Geometry: final body of the model. Coordinates: model frame, mm. A direction names the side the tool comes from. Round coordinates to 2 decimals unless told otherwise and drop trailing zeros. Loops run counter-clockwise (first coordinate to the right, second up) from the corner with the lowest first, then second, coordinate; pieces in that order, holes last. Notation, with made-up numbers: (26, 14) -> (30, 14) arc R17 ccw to (30, 20) -> close; hole circle Ø1 at (25.25, 14). An arc over 180 degrees is marked (long way). Answer in a Markdown table with one row per item.
```python
from build123d import *

# Parameters (mm, degrees)
F0_R     = 12.7
F0_R_2   = 9.525
F1_DEPTH = 50.8
F2_R     = 12.7
F4_DEPTH = 25.4
F3_R     = 9.525
F5_DEPTH = 25.4


with BuildPart() as f1:
    # F0 (on Front) → F1 (new body)
    with BuildSketch(Plane.XZ):
        Circle(F0_R)
        Circle(F0_R_2, mode=Mode.SUBTRACT)
    extrude(amount=F1_DEPTH)

    # F2 (on Right) → F4 (join)
    with BuildSketch(Plane.YZ):
        with Locations((-25.363049, 0)):
            Circle(F2_R)
    extrude(amount=F4_DEPTH)

    # F3 (on Right) → F5 (cut)
    with BuildSketch(Plane.YZ):
        with Locations((-25.363049, 0)):
            Circle(F3_R)
    extrude(amount=F5_DEPTH, mode=Mode.SUBTRACT)


solid = f1.part
```
Item 1: Section query B-B, the plane y = -14. Output: boundary loops of the cut face in (x, z) (3 decimals).
Ans:
| item | result |
|---|---|
| outline | (11.363, -5.672) -> (25.4, -5.672) -> (25.4, 5.672) -> (11.363, 5.672) arc R12.7 ccw (long way) to start; hole (0, -5.672) -> (0, 5.672) -> (7.652, 5.672) arc R9.525 ccw (long way) to (7.652, -5.672) -> close |
Item 2: Set-up query: faces 1 (the flat face through (5, -50.8, 9)), 2 (the cylindrical face through (-9.516, -25.044, 0.419)), 3 (the flat face through (5, 0, 9)), 4 (the cylindrical face through (15.34, -13.25, 3.81)), 5 (the flat face through (0, -35, 1)). Return all of +Z, -Z, +X, -X, +Y, -Y with unobstructed straight access to the full face (end or side cutting, diameter ignored); none if empty.
Ans:
| item | result |
|---|---|
| face 1 | +Z, -Z, +X, -X, -Y |
| face 2 | none |
| face 3 | +Z, -Z, +X, -X, +Y |
| face 4 | +X |
| face 5 | +Y, -Y |
Item 3: Section query C-C, the plane x = 10.5. Output: boundary loops of the cut face in (y, z) (3 decimals), and give its area (3 significant figures).
Ans:
| item | result |
|---|---|
| outline | (-50.8, -7.144) -> (-35.863, -7.144) arc R12.7 ccw to (-14.863, -7.144) -> (0, -7.144) -> (0, 7.144) -> (-14.863, 7.144) arc R12.7 ccw to (-35.863, 7.144) -> (-50.8, 7.144) -> close; hole circle Ø19.05 at (-25.363, 0) |
| area | 605 mm2 |
Item 4: Mould query, pull axis X, two halves, no side actions, for faces 6 (the flat face through (25.4, -23.5, 9.5)), 7 (the cylindrical face through (3.637, -38.062, 0.151)), 8 (the cylindrical face through (-12.688, -25.044, 0.558)). Classes: released by +X, released by -X, zero draft, split by the parting line, or undercut.
Ans:
| item | result |
|---|---|
| face 6 | released by +X |
| face 7 | undercut |
| face 8 | split by the parting line |
Item 5: Section query A-A, the plane z = 0. Output: boundary loops of the cut face in (x, y) (3 decimals), and give its area (3 significant figures).
Ans:
| item | result |
|---|---|
| outline | (-12.7, -50.8) -> (-9.525, -50.8) -> (-9.525, 0) -> (-12.7, 0) -> close; (0, -38.063) -> (9.525, -38.063) -> (9.525, -50.8) -> (12.7, -50.8) -> (12.7, -38.063) -> (25.4, -38.063) -> (25.4, -34.888) -> (0, -34.888) -> close; (0, -15.838) -> (25.4, -15.838) -> (25.4, -12.663) -> (12.7, -12.663) -> (12.7, 0) -> (9.525, 0) -> (9.525, -12.663) -> (0, -12.663) -> close |
| area | 403 mm2 |
Item 6: First-contact query: P1, Ø4, axis at y = -31.5, z = -2.5, coming from the -X side; P2, Ø12, axis at x = 19.5, z = 0, coming from the -Y side; P3, Ø8, axis at x = 18.5, y = -36.5, coming from the +Z side. Flat tips, straight axial feed; report the tip coordinate or a pass-through.
Ans:
| item | result |
|---|---|
| P1 | x = -12.69 |
| P2 | y = -38.06 |
| P3 | z = 10.5 |
Item 7: Ray query, L1, parallel to Y at x = 16.5, z = 0; L2, parallel to Z at x = -0.5, y = -18; L3, parallel to X at y = -47.5, z = -2.75. Return the intervals inside material, ascending.
Ans:
| item | result |
|---|---|
| L1 | -38.06 to -34.89, -15.84 to -12.66 |
| L2 | -12.69 to -9.51, 9.51 to 12.69 |
| L3 | -12.4 to -9.12, 9.12 to 12.4 |
Item 8: Section query D-D, the plane y = -28. Output: boundary loops of the cut face in (x, z) (3 decimals).
Ans:
| item | result |
|---|---|
| outline | (0, -9.525) arc R9.525 cw to (0, 9.525) -> (0, 9.153) -> (25.4, 9.153) -> (25.4, 12.423) -> (2.637, 12.423) arc R12.7 ccw (long way) to (2.637, -12.423) -> (25.4, -12.423) -> (25.4, -9.153) -> (0, -9.153) -> close |
